The model under review builds one solid part; all positions refer to its coordinate system, in mm. A direction names the side the tool comes from. Give positions to 0.01 mm unless a question says otherwise; leave off trailing zeros. Order: outer loops, then holes, each group sorted by start corner. A loop starts at its lowest first (then second) coordinate and runs counter-clockwise, first axis right, second up.
```python
from build123d import *

# Parameters (mm, degrees)
F0_W     = 101.6
F0_H     = 81.743848
F1_DEPTH = 91.948
F2_R     = 5.08
F3_R     = 50.736946
F4_DEPTH = 40.872924


with BuildPart() as f1:
    # F0 (on Front) → F1 (new body)
    with BuildSketch(Plane.XZ):
        Rectangle(F0_W, F0_H)
    extrude(amount=F1_DEPTH)

    # F2
    f2_edges = [f1.edges().sort_by_distance(p)[0] for p in [
        (-50.8, -91.948, 0),
        (0, -91.948, -40.871924),
        (50.8, -91.948, 0),
        (0, -91.948, 40.871924),
    ]]
    fillet(f2_edges, radius=F2_R)

    # F3 (on Top) → F4 (cut, through all)
    with BuildSketch(Plane.XY):
        Circle(F3_R)
    extrude(amount=-F4_DEPTH, mode=Mode.SUBTRACT)


solid = f1.part
```
Item 1: Take a section at B-B (x = 0). Give the boundary of the cut face in (y, z).
Values found:
outline: (-91.95, -35.79) arc R5.08 ccw to (-86.87, -40.87) - (-50.74, -40.87) - (-50.74, 0) - (0, 0) - (0, 40.87) - (-86.87, 40.87) arc R5.08 ccw to (-91.95, 35.79) - close
Item 2: For faces 1 (the flat face through (-1, -19, 0)), 2 (the cylindrical face through (-49.35, -90.42, 0.57)), list the 3-axis set-ups (+Z, -Z, +X, -X, +Y, -Y) from which the entire face can be reached by the end or side of a thin tool; tool diameter is ignored.
Values found:
face 1: -Z, +Y
face 2: +Z, -Z, -X, -Y
Item 3: Take a section at A-A (z = -33.5). Give the boundary of the cut face in (x, y), and give its area (3 significant figures).
Values found:
outline: (-50.8, -86.87) arc R5.08 ccw to (-45.72, -91.95) - (45.72, -91.95) arc R5.08 ccw to (50.8, -86.87) - (50.8, 0) - (50.74, 0) arc R50.74 cw to (-50.74, 0) - (-50.8, 0) - close
area: 5,290 mm2
Item 4: Draft analysis for pull direction X (two halves, no side actions). For faces 3 (the flat face through (50.8, -43, -1)), 4 (the cylindrical face through (-1.116, -50.725, -20.15)), 5 (the flat face through (-1, -43, 40.872)), state which applies: released by +X, released by -X, zero draft, split by the parting line, or undercut.
Values found:
face 3: released by +X
face 4: undercut
face 5: zero draft
Item 5: For line 1 (Z direction, x = 38, y = -11.5); line 2 (X direction, y = -37.5, z = -29); line 3 (X direction, y = -20, z = -27.5), list the stretches that pass through material, from the lowest coordinate up.
Values found:
line 1: z = 0 to 40.87
line 2: x = -50.8 to -34.18, 34.18 to 50.8
line 3: x = -50.8 to -46.63, 46.63 to 50.8
